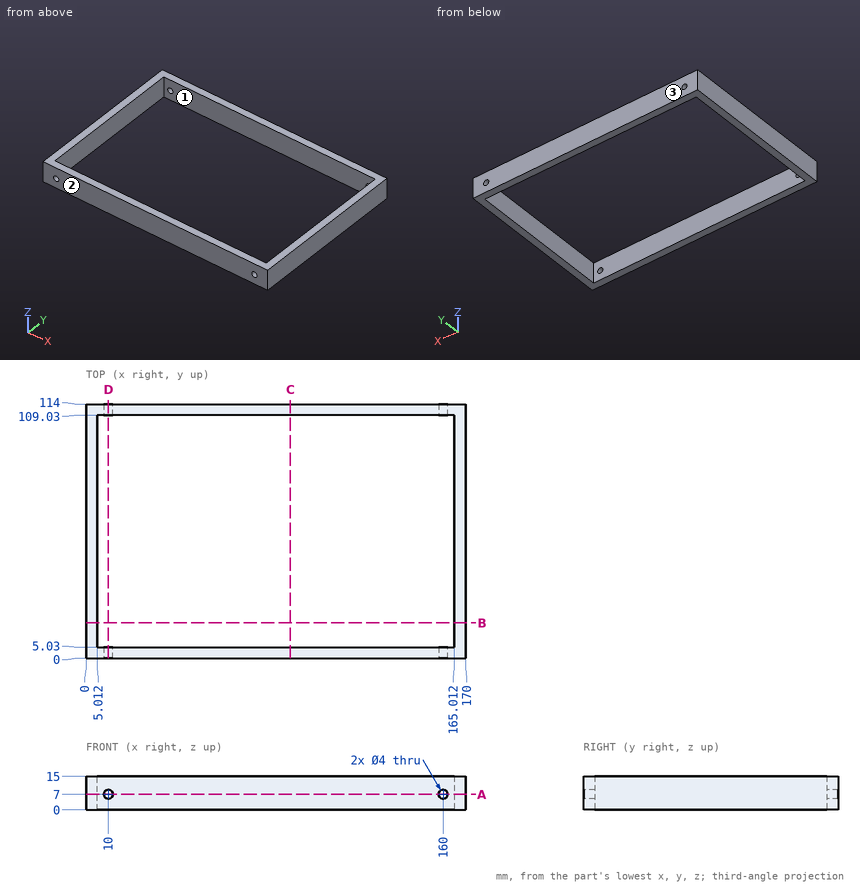
Answer from the drawing. Dimensions are ordinates in mm from the lowest x, y and z of the part. Coordinates: 2 decimals unless noted, no trailing zeros. Order: outer loops, then holes, each group sorted by start corner. A loop starts at its lowest first (then second) coordinate and runs counter-clockwise, first axis right, second up. Notation, with made-up numbers: (86, 76) - (145, 76) arc R18 ccw to (145, 89) - close; hole circle Ø2 at (45.25, 72). An arc over 180 degrees is marked (long way). Answer as a JSON object with one key per item and string values. Group by question number.
Item 1: Section A-A (z = 7) is taken. Give the vertices of the cut face in (x, y).
Item 2: Consider probe 1 along X at (y, z) = (1.75, 7); probe 2 along X at (y, z) = (8.5, 12); probe 3 along Y at (x, z) = (115.5, 13.5). Determine where each line is inside the solid, lowest interval first. Write a range as from..to.
Item 3: A flat-ended cylindrical pin translates along its axis: P1, Ø2.5, axis at x = 10, z = 7, coming from the -Y side. Find the tip coordinate at first contact, or state that the pin passes through.
Item 4: Section B-B (y = 16) is taken. Give the vertices of the cut face in (x, z), plus the area to 3 significant figures.
Item 5: Section D-D (x = 10) is taken. Give the vertices of the cut face in (y, z), plus the area to 3 significant figures.
Item 6: The mould has two halves that part along Y. Classify the marked faces 1, 2 and 3: +Y half, -Y half, draft (parallel to the pull), parting line (faces both ways), or undercut.
Item 7: Section C-C (x = 91.5) is taken. Give the vertices of the cut face in (y, z).
Results are:
{
 "1": {"outline": "(0, 0) - (8, 0) - (8, 5.03) - (5.01, 5.03) - (5.01, 109.03) - (8, 109.03) - (8, 114) - (0, 114) - close; (12, 0) - (158, 0) - (158, 5.03) - (12, 5.03) - close; (12, 109.03) - (158, 109.03) - (158, 114) - (12, 114) - close; (162, 0) - (170, 0) - (170, 114) - (162, 114) - (162, 109.03) - (165.01, 109.03) - (165.01, 5.03) - (162, 5.03) - close"},
 "2": {"probe 1": "x = 0..8, 12..158, 162..170", "probe 2": "x = 0..5.01, 165.01..170", "probe 3": "y = 0..5.03, 109.03..114"},
 "3": {"P1": "passes through"},
 "4": {"outline": "(0, 0) - (5.01, 0) - (5.01, 15) - (0, 15) - close; (165.01, 0) - (170, 0) - (170, 15) - (165.01, 15) - close", "area": "150 mm^2"},
 "5": {"outline": "(0, 0) - (5.03, 0) - (5.03, 5) - (0, 5) - close; (0, 9) - (5.03, 9) - (5.03, 15) - (0, 15) - close; (109.03, 0) - (114, 0) - (114, 5) - (109.03, 5) - close; (109.03, 9) - (114, 9) - (114, 15) - (109.03, 15) - close", "area": "110 mm^2"},
 "6": {"face 1": "undercut", "face 2": "-Y half", "face 3": "+Y half"},
 "7": {"outline": "(0, 0) - (5.03, 0) - (5.03, 15) - (0, 15) - close; (109.03, 0) - (114, 0) - (114, 15) - (109.03, 15) - close"}
}
